from build123d import *

# Parameters (mm, degrees)
F0_R     = 19
F1_DEPTH = 18


with BuildPart() as f1:
    # F0 (on Top) → F1 (new body)
    with BuildSketch(Plane.XY):
        with BuildLine():
            Line((79.915271, 225), (-595.084729, 225))
            ThreePointArc((-595.084729, 225), (-665.795407, 195.710678), (-695.084729, 125))
            Line((-695.084729, 125), (-695.084729, -125))
            ThreePointArc((-695.084729, -125), (-665.795407, -195.710678), (-595.084729, -225))
            Line((-595.084729, -225), (79.915271, -225))
            ThreePointArc((79.915271, -225), (150.625949, -195.710678), (179.915271, -125))
            Line((179.915271, -125), (179.915271, 125))
            ThreePointArc((179.915271, 125), (150.625949, 195.710678), (79.915271, 225))
        make_face()
        with Locations((-505.084729, 0)):
            Circle(F0_R, mode=Mode.SUBTRACT)
        Circle(F0_R, mode=Mode.SUBTRACT)
    extrude(amount=F1_DEPTH)


solid = f1.part
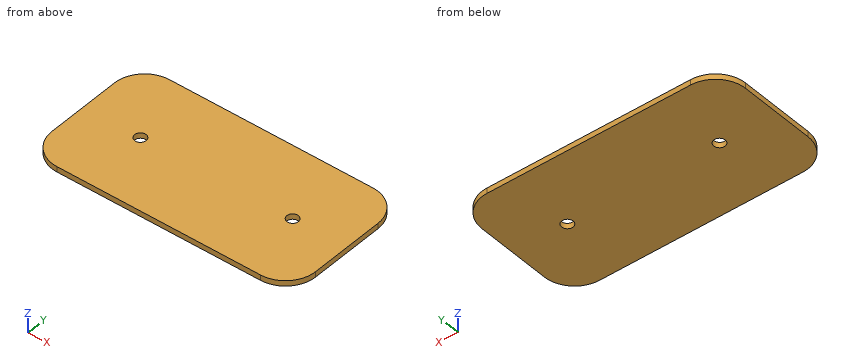
CAD build for the part. Positions are in the model's coordinates, mm. Coordinates: 2 decimals unless noted, no trailing zeros. Order: outer loops, then holes, each group sorted by start corner. A loop starts at its lowest first (then second) coordinate and runs counter-clockwise, first axis right, second up.
Item 1: Band-saw the part on B-B on x = 0. List the corners of the cut face in (y, z).
Check sheet entries:
outline: (-225, 0) - (-19, 0) - (-19, 18) - (-225, 18) - close; (19, 0) - (225, 0) - (225, 18) - (19, 18) - close
Item 2: Band-saw the part on A-A on y = 0. List the corners of the cut face in (x, z).
Check sheet entries:
outline: (-695.08, 0) - (-524.08, 0) - (-524.08, 18) - (-695.08, 18) - close; (-486.08, 0) - (-19, 0) - (-19, 18) - (-486.08, 18) - close; (19, 0) - (179.92, 0) - (179.92, 18) - (19, 18) - close
Item 3: Drill centre lines: L1, parallel to Y at x = 0, z = 8.75; L2, parallel to Y at x = -17, z = 3.5; L3, parallel to X at y = 135.5, z = 6.75. Where is each one in solid material? Low to high.
Check sheet entries:
L1: y = -225 to -19, 19 to 225
L2: y = -225 to -8.49, 8.49 to 225
L3: x = -694.53 to 179.36
Item 4: Band-saw the part on C-C on z = 5. List the corners of the cut face in (x, y).
Check sheet entries:
outline: (-695.08, -125) arc R100 ccw to (-595.08, -225) - (79.92, -225) arc R100 ccw to (179.92, -125) - (179.92, 125) arc R100 ccw to (79.92, 225) - (-595.08, 225) arc R100 ccw to (-695.08, 125) - close; hole circle Ø38 at (-505.08, 0); hole circle Ø38 at (0, 0)
Item 5: Pin check, flat tip, straight feed: pin 1 Ø2 at (x, y) = (-376, 144.5) entering from -Z. Stop position of the tip, or through.
Check sheet entries:
pin 1: stops at z = 0
